Can you work these out from the model? Positions are in its coordinate system, mm. A direction names the side the tool comes from. Give positions to 0.01 mm unless a question says otherwise; leave off trailing zeros. Write each loop counter-clockwise with the first axis right and the second up, starting at its lowest first coordinate (ties: lowest second). Pieces come first, ordered by that corner, then holes.
from build123d import *

# Parameters (mm, degrees)
SKETCH2_R           = 10.2
BOSS_EXTRUDE1_DEPTH = 12.9
SKETCH4_R           = 11.9
SKETCH4_R_2         = 10.2
BOSS_EXTRUDE2_DEPTH = 19.8


with BuildPart() as part:
    # Sketch1 → Revolve1 (revolve)
    with BuildSketch(Plane(origin=(0, 0, 0), x_dir=(0, 0, -1), z_dir=(1, 0, 0))):
        Polygon((0, 10.2), (0, 18.3), (-3.5, 18.3), (-8.17653718, 10.2), align=None)
    revolve(axis=Axis((0, 0, 27.758529938), (0, 0, -1)))

    # Sketch2 → Boss-Extrude1 (add)
    with BuildSketch(Plane.XY):
        with BuildLine():
            Line((18.071063426, 0.5), (9.468544415, 15.4))
            ThreePointArc((9.468544415, 15.4), (9.102519011, 15.766025404), (8.602519011, 15.9))
            Line((8.602519011, 15.9), (-8.602519011, 15.9))
            ThreePointArc((-8.602519011, 15.9), (-9.102519011, 15.766025404), (-9.468544415, 15.4))
            Line((-9.468544415, 15.4), (-18.071063426, 0.5))
            ThreePointArc((-18.071063426, 0.5), (-18.205038022, 0), (-18.071063426, -0.5))
            Line((-18.071063426, -0.5), (-9.468544415, -15.4))
            ThreePointArc((-9.468544415, -15.4), (-9.102519011, -15.766025404), (-8.602519011, -15.9))
            Line((-8.602519011, -15.9), (8.602519011, -15.9))
            ThreePointArc((8.602519011, -15.9), (9.102519011, -15.766025404), (9.468544415, -15.4))
            Line((9.468544415, -15.4), (18.071063426, -0.5))
            ThreePointArc((18.071063426, -0.5), (18.205038022, 0), (18.071063426, 0.5))
        make_face()
        Circle(SKETCH2_R, mode=Mode.SUBTRACT)
    extrude(amount=BOSS_EXTRUDE1_DEPTH)

    # Sketch3 → Cut-Revolve2 (revolve, cut)
    with BuildSketch(Plane(origin=(0, 0, 0), x_dir=(0, 0, -1), z_dir=(1, 0, 0))):
        Polygon((-11.414359354, 18.3), (-21.97986928, 0), (-22.588162692, 0), (-22.588162692, 18.3), align=None)
    revolve(axis=Axis((0, 0, 0), (0, 0, 1)), mode=Mode.SUBTRACT)

    # Sketch4 → Boss-Extrude2 (add)
    with BuildSketch(Plane.XY):
        Circle(SKETCH4_R)
        Circle(SKETCH4_R_2, mode=Mode.SUBTRACT)
    extrude(amount=BOSS_EXTRUDE2_DEPTH)


solid = part.part
(1) Imagine slicing it at D-D, the plane z = 17.5. Write out the boundary of the cut face in (x, y).
Returned:
outline: circle Ø23.8 at (0, 0); hole circle Ø20.4 at (0, 0)
(2) Imagine slicing it at B-B, the plane z = 7.5. Write out the boundary of the cut face in (x, y).
Returned:
outline: (-18.07, -0.5) - (-9.47, -15.4) arc R1 ccw to (-8.6, -15.9) - (8.6, -15.9) arc R1 ccw to (9.47, -15.4) - (18.07, -0.5) arc R1 ccw to (18.07, 0.5) - (9.47, 15.4) arc R1 ccw to (8.6, 15.9) - (-8.6, 15.9) arc R1 ccw to (-9.47, 15.4) - (-18.07, 0.5) arc R1 ccw to start; hole circle Ø20.4 at (0, 0)
(3) Imagine slicing it at A-A, the plane x = 0. Write out the boundary of the cut face in (y, z), plus the area to 3 significant figures.
Returned:
outline: (-18.3, 0) - (-10.2, 0) - (-10.2, 19.8) - (-11.9, 19.8) - (-11.9, 12.9) - (-15.73, 12.9) - (-15.9, 12.8) - (-15.9, 4.89) - (-18.3, 3.5) - close; (10.2, 0) - (18.3, 0) - (18.3, 3.5) - (15.9, 4.89) - (15.9, 12.8) - (15.73, 12.9) - (11.9, 12.9) - (11.9, 19.8) - (10.2, 19.8) - close
area: 191 mm2
(4) If I drill on L1, parallel to Y at x = 0, z = 5.75; L2, parallel to Y at x = 0, z = 16; L3, parallel to X at y = 7, z = 5, over which ranges is the centre line in solid material (lowest first)?
Returned:
L1: y = -15.9 to -10.2, 10.2 to 15.9
L2: y = -11.9 to -10.2, 10.2 to 11.9
L3: x = -14.32 to -7.42, 7.42 to 14.32
(5) If we mould it in two halves opening along Y, with no side actions, what happens to faces 1 (the face through (0, 15.9, 8)), 2 (the face through (-2, 12, 12.9)), 3 (the face through (4.707, -9.049, 9.761))? For each: +Y half, -Y half, draft (parallel to the pull), parting line (faces both ways), or undercut.
Returned:
face 1: +Y half
face 2: draft
face 3: undercut
(6) For faces 4 (the face through (13.83, 7.846, 8.15)), 5 (the face through (13.71, -8.05, 8.15)), 6 (the face through (18.205, -0.007, 7.493)), 7 (the face through (-9.096, 15.77, 7.493)), which set-ups out of +Z, -Z, +X, -X, +Y, -Y let a thin tool reach every point of the face, with its end or its side?
Returned:
face 4: +Z, +X, +Y
face 5: +Z, +X, -Y
face 6: +Z, +X
face 7: +Z, -X, +Y
(7) Imagine slicing it at C-C, the plane y = 0. Write out the boundary of the cut face in (x, z), plus the area to 3 significant figures.
Returned:
outline: (-18.3, 0) - (-10.2, 0) - (-10.2, 19.8) - (-11.9, 19.8) - (-11.9, 12.9) - (-15.73, 12.9) - (-18.21, 11.47) - (-18.21, 3.55) - (-18.3, 3.5) - close; (10.2, 0) - (18.3, 0) - (18.3, 3.5) - (18.21, 3.55) - (18.21, 11.47) - (15.73, 12.9) - (11.9, 12.9) - (11.9, 19.8) - (10.2, 19.8) - close
area: 227 mm2
(8) Will these pins go through, and if not, where does the flat tip stop? P1, Ø2, axis at x = 12, z = 6.5, coming from the -Y side; P2, Ø3, axis at x = -0.5, z = 7, coming from the -Y side; P3, Ø10, axis at x = 3.5, z = 9.5, coming from the +Y side.
Returned:
P1: stops at y = -12.75
P2: stops at y = -15.9
P3: stops at y = 16.25
